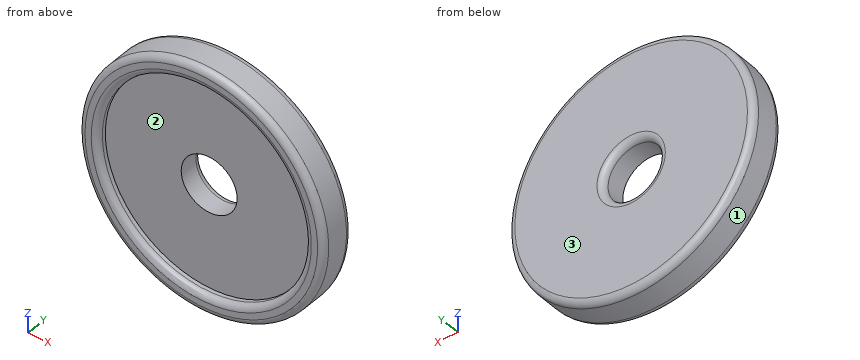
```python
from build123d import *

# Parameters (mm, degrees)
FILLET1_R = 0.5


with BuildPart() as part:
    # Sketch1 → Revolve1 (revolve)
    with BuildSketch(Plane.XY):
        Polygon((-2.2479, 0), (-2.2479, 2), (-9.8479, 2), (-9.8479, -0.8), (-8.3479, -0.8), (-8.3479, 0), align=None)
    revolve(axis=Axis((0, 0, 0), (0, 1, 0)))

    # Fillet1
    fillet1_edges = [part.edges().sort_by_distance(p)[0] for p in [
        (8.3479, -0.8, 0),
        (9.8479, -0.8, 0),
        (9.8479, 2, 0),
        (2.2479, 2, 0),
    ]]
    fillet(fillet1_edges, radius=FILLET1_R)


solid = part.part
```
Part model, mm, in its own coordinate system. Face numbers are marked on the shaded views. Round coordinates to 2 decimals unless told otherwise and drop trailing zeros. Write each loop counter-clockwise with the first axis right and the second up, starting at its lowest first coordinate (ties: lowest second). Pieces come first, ordered by that corner, then holes. Notation, with made-up numbers: M -17,84 L 29,84 A19 ccw 29,104 Z; hole C 61.5,35 d7. An arc over 180 degrees is marked long. Answer as CSV lines item,"result". Start each with the question number.
1) Mould opens along X. For the marked faces 1, 2 and 3 say: +X half, -X half, draft (parallel to the pull), parting line (faces both ways), or undercut.
2) Band-saw the part on B-B (y = 0.5). List the corners of the cut face in (x, z).
3) Drill centre lines: L1, parallel to Z at x = 0, y = 1.2; L2, parallel to Z at x = 0, y = -0.2; L3, parallel to Y at x = -8.75, z = -0.75. Where is each one in solid material? Low to high.
4) Band-saw the part on A-A (x = 0). List the corners of the cut face in (y, z), then the cut area to 3 significant figures.
5) Drop flat-ended pins along their axis: pin 1 (5 mm diameter, centred on x = 1, z = 0.5, fed in from -Y); pin 2 (4 mm diameter, centred on x = 0, z = 0, fed in from -Y). Give the stop position or say it passes through.
Worked out:
1,face 1,"parting line"
1,face 2,"undercut"
1,face 3,"draft"
2,outline,"C 0,0 d19.7; hole C 0,0 d4.5"
3,L1,"-9.85 to -2.25, 2.25 to 9.85"
3,L2,"-9.85 to -8.35, 8.35 to 9.85"
3,L3,"-0.8 to 2"
4,outline,"M -0.8,-9.35 A0.5 ccw -0.3,-9.85 L 1.5,-9.85 A0.5 ccw 2,-9.35 L 2,-2.75 A0.5 ccw 1.5,-2.25 L 0,-2.25 L 0,-8.35 L -0.3,-8.35 A0.5 ccw -0.8,-8.85 Z; M -0.8,8.85 A0.5 ccw -0.3,8.35 L 0,8.35 L 0,2.25 L 1.5,2.25 A0.5 ccw 2,2.75 L 2,9.35 A0.5 ccw 1.5,9.85 L -0.3,9.85 A0.5 ccw -0.8,9.35 Z"
4,area,"32.4 mm²"
5,pin 1,"y = 0"
5,pin 2,"through"
